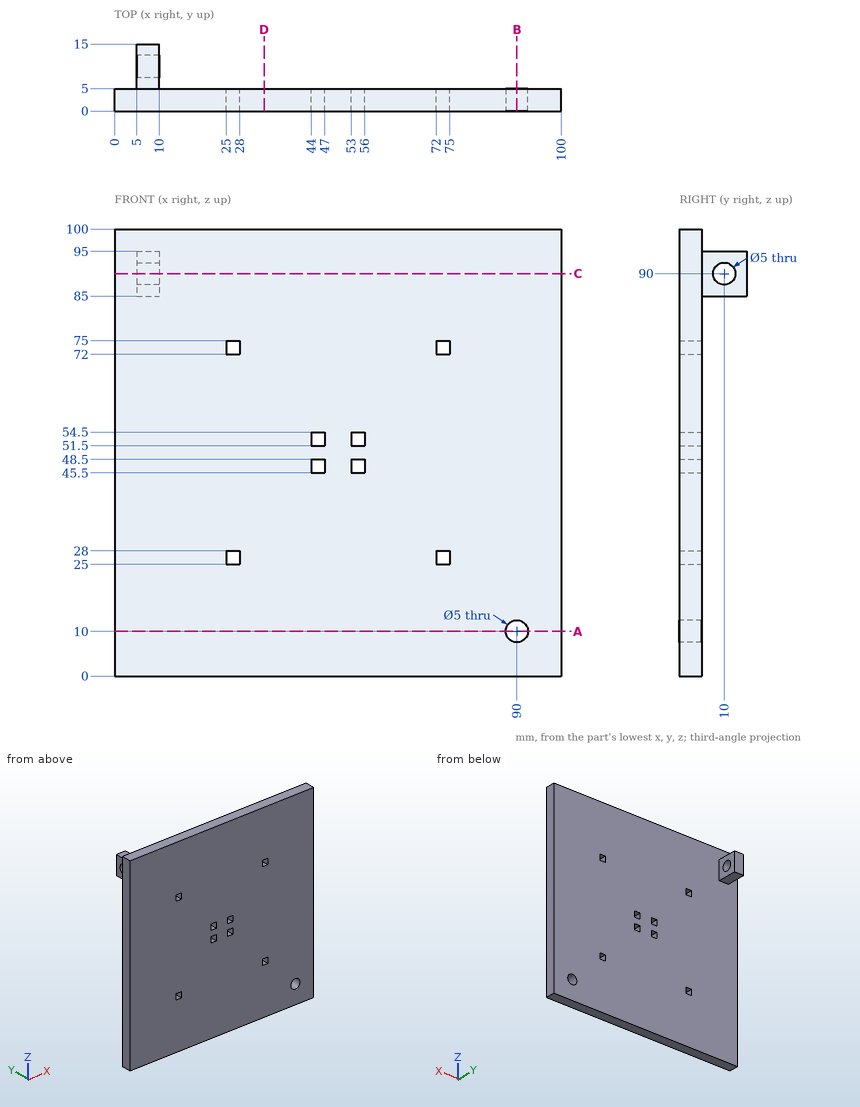
Drawing for the job (mm, zero at the part's lowest x, y, z). Round coordinates to 2 decimals unless told otherwise and drop trailing zeros. Write each loop counter-clockwise with the first axis right and the second up, starting at its lowest first coordinate (ties: lowest second). Pieces come first, ordered by that corner, then holes. Notation, with made-up numbers: M 3.5,-6.75 L 60.5,-6.75 A24 ccw 60.5,3.25 Z; hole C 87.5,-19 d3. An arc over 180 degrees is marked long. One line per question, with ' | ' between items.
1. Cut at B-B on x = 90. Write the cut outline in (y, z), and give its area (3 significant figures).
Working result:
outline: M 0,0 L 5,0 L 5,7.5 L 0,7.5 Z; M 0,12.5 L 5,12.5 L 5,100 L 0,100 Z | area: 475 mm2
2. Cut at D-D on x = 33.5. Write the cut outline in (y, z), and give its area (3 significant figures).
Working result:
outline: M 0,0 L 5,0 L 5,100 L 0,100 Z | area: 500 mm2
3. Cut at A-A on z = 10. Write the cut outline in (x, y).
Working result:
outline: M 0,0 L 87.5,0 L 87.5,5 L 0,5 Z; M 92.5,0 L 100,0 L 100,5 L 92.5,5 Z
4. Pin check, flat tips, straight feed: pin 1 Ø10 at (x, z) = (69, 61.5) entering from -Y; pin 2 Ø8 at (x, z) = (22, 51.5) entering from +Y; pin 3 Ø5 at (y, z) = (12, 92) entering from -X. Stop position of each tip, or through.
Working result:
pin 1: y = 0 | pin 2: y = 5 | pin 3: x = 5
5. Probe L1, parallel to Y at x = 6.6, z = 90; L2, parallel to Z at x = 90, y = 1.05; L3, parallel to Y at x = 30, z = 20.5. List the from-to ranges inside material, lowest first. Write a range as from..to.
Working result:
L1: 0..7.5, 12.5..15 | L2: 0..7.5, 12.5..100 | L3: 0..5
6. Cut at C-C on z = 90. Write the cut outline in (x, y), and give its area (3 significant figures).
Working result:
outline: M 0,0 L 100,0 L 100,5 L 10,5 L 10,7.5 L 5,7.5 L 5,5 L 0,5 Z; M 5,12.5 L 10,12.5 L 10,15 L 5,15 Z | area: 525 mm2
